Here's how the part is built. I have some questions about the finished solid (model axes, mm). Round coordinates to 2 decimals unless told otherwise and drop trailing zeros. Loops run counter-clockwise (first coordinate to the right, second up) from the corner with the lowest first, then second, coordinate; pieces in that order, holes last. Notation, with made-up numbers: (78.25, 47.5) - (108.25, 47.5) arc R21 ccw to (108.25, 68.5) - close; hole circle Ø5 at (72.25, 44). An arc over 180 degrees is marked (long way). Return JSON: item names as keys, results as strings. Group by question number.
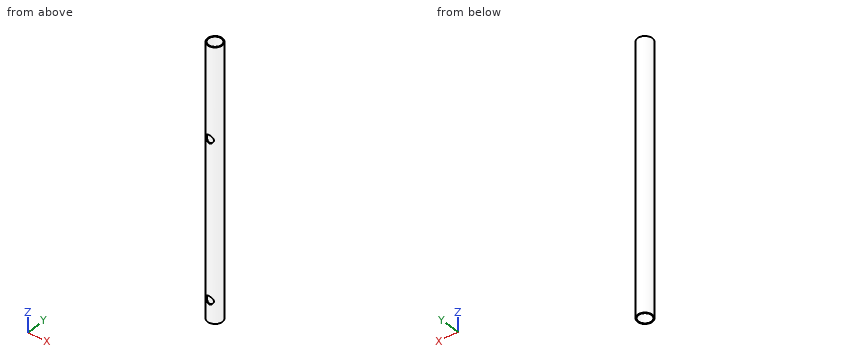
```python
from build123d import *

# Parameters (mm, degrees)
F0_R     = 16.75
F1_DEPTH = 609.6
F2_R     = 14.75
F3_DEPTH = 609.6
F4_R     = 9
F6_DEPTH = 25
F5_R     = 9
F7_DEPTH = 25


with BuildPart() as f1:
    # F0 (on Top) → F1 (new body)
    with BuildSketch(Plane.XY):
        Circle(F0_R)
    extrude(amount=-F1_DEPTH)

    # F2 (on Top) → F3 (cut)
    with BuildSketch(Plane.XY):
        Circle(F2_R)
    extrude(amount=-F3_DEPTH, mode=Mode.SUBTRACT)

    # F4 (on Front) → F6 (cut)
    with BuildSketch(Plane.XZ):
        with Locations((0, -204.8)):
            Circle(F4_R)
    extrude(amount=F6_DEPTH, mode=Mode.SUBTRACT)

    # F5 (on Front) → F7 (cut)
    with BuildSketch(Plane.XZ):
        with Locations((0, -559.8)):
            Circle(F5_R)
    extrude(amount=F7_DEPTH, mode=Mode.SUBTRACT)


solid = f1.part
```
Q1. Please list where these lines run through material, in increasing order: line 1 (Z direction, x = 0, y = -15.45); line 2 (X direction, y = 0.5, z = -296); line 3 (Y direction, x = -1, z = -305.5).
Q2. Will these pins go through, and if not, where does the flat tip stop? pin 1 Ø1 at (x, z) = (-3, -531.5) entering from +Y; pin 2 Ø1.5 at (y, z) = (9.5, -520) entering from -X; pin 3 Ø17.5 at (x, y) = (0, 0) entering from -Z; pin 4 Ø8 at (y, z) = (13, -279.5) entering from +X.
Q3. Imagine slicing it at B-B, the plane x = 0. List the corners of the cut face in (y, z) for me, and give its area (3 significant figures).
Q4. Imagine slicing it at C-C, the plane z = -381. List the corners of the cut face in (x, y) for me, and give its area (3 significant figures).
Q5. Imagine slicing it at A-A, the plane y = 0. List the corners of the cut face in (x, z) for me, and give its area (3 significant figures).
Q6. Imagine slicing it at D-D, the plane z = -559.8. List the corners of the cut face in (x, y) for me, and give its area (3 significant figures).
Output values:
{
 "1": {"line 1": "z = -609.6 to -568.8, -550.8 to -213.8, -195.8 to 0", "line 2": "x = -16.74 to -14.74, 14.74 to 16.74", "line 3": "y = -16.72 to -14.72, 14.72 to 16.72"},
 "2": {"pin 1": "stops at y = 16.56", "pin 2": "stops at x = -14.28", "pin 3": "passes through", "pin 4": "stops at x = 14.13"},
 "3": {"outline": "(-16.75, -609.6) - (-14.75, -609.6) - (-14.75, -568.8) - (-16.75, -568.8) - close; (-16.75, -550.8) - (-14.75, -550.8) - (-14.75, -213.8) - (-16.75, -213.8) - close; (-16.75, -195.8) - (-14.75, -195.8) - (-14.75, 0) - (-16.75, 0) - close; (14.75, -609.6) - (16.75, -609.6) - (16.75, 0) - (14.75, 0) - close", "area": "2,370 mm^2"},
 "4": {"outline": "circle Ø33.5 at (0, 0); hole circle Ø29.5 at (0, 0)", "area": "198 mm^2"},
 "5": {"outline": "(-16.75, -609.6) - (-14.75, -609.6) - (-14.75, 0) - (-16.75, 0) - close; (14.75, -609.6) - (16.75, -609.6) - (16.75, 0) - (14.75, 0) - close", "area": "2,440 mm^2"},
 "6": {"outline": "(-9, -14.13) - (-9, -11.69) arc R14.75 cw (long way) to (9, -11.69) - (9, -14.13) arc R16.75 ccw (long way) to start", "area": "160 mm^2"}
}
